from build123d import *

# Parameters (mm, degrees)
F0_W     = 2
F0_H     = 78
F1_DEPTH = 25
F0_W_2   = 16
F2_DEPTH = 2
F3_W     = 45.6874087788
F3_H     = 12.5
F4_DEPTH = 10
F7_DEPTH = 78
F8_DEPTH = 78


# Not quite as in the source:
# - a feature names something its author has since deleted; it is built from what else it names


with BuildPart() as f1:
    # F0 (on Top) → F1 (new body)
    with BuildSketch(Plane.XY):
        with Locations((9, 0)):
            Rectangle(F0_W, F0_H)
    extrude(amount=F1_DEPTH)



with BuildPart() as f1b:
    # F0 (on Top) → F1, piece 2 (new body)
    with BuildSketch(Plane.XY):
        with Locations((-9, 0)):
            Rectangle(F0_W, F0_H)
    extrude(amount=F1_DEPTH)


with BuildPart() as f1_1:
    add(f1.part)

    add(f1b.part)  # F2 merges F1b
    # F0 (on Top) → F2 (join)
    with BuildSketch(Plane.XY):
        with Locations((9, 0)):
            Rectangle(F0_W, F0_H)
        Rectangle(F0_W_2, F0_H)
        with Locations((-9, 0)):
            Rectangle(F0_W, F0_H)
    extrude(amount=F2_DEPTH)

    # F3 (on face) → F4 (cut)
    with BuildSketch(Plane(origin=(-10, 0, 0), x_dir=(0, -1, 0), z_dir=(-1, 0, 0))):
        with Locations((16.1562956106, 18.75)):
            Rectangle(F3_W, F3_H)
    extrude(amount=-F4_DEPTH, mode=Mode.SUBTRACT)

    # F6 (on face) → F7 (join)
    with BuildSketch(Plane(origin=(0, 39, 0), x_dir=(-1, 0, 0), z_dir=(0, 1, 0))):
        with BuildLine():
            ThreePointArc((-10, 7.8135579824), (-11.356996059, 3.1753555196), (-15, 0))
            Line((-15, 0), (-10, 0))
            Line((-10, 0), (-10, 7.8135579824))
        make_face()
    extrude(amount=-F7_DEPTH)

    # F5 (on face) → F8 (join)
    with BuildSketch(Plane(origin=(0, 39, 0), x_dir=(-1, 0, 0), z_dir=(0, 1, 0))):
        with BuildLine():
            Line((10, 0), (15, 0))
            ThreePointArc((15, 0), (11.360255444, 3.0951443467), (10, 7.6752495952))
            Line((10, 7.6752495952), (10, 0))
        make_face()
    extrude(amount=-F8_DEPTH)


solid = f1_1.part
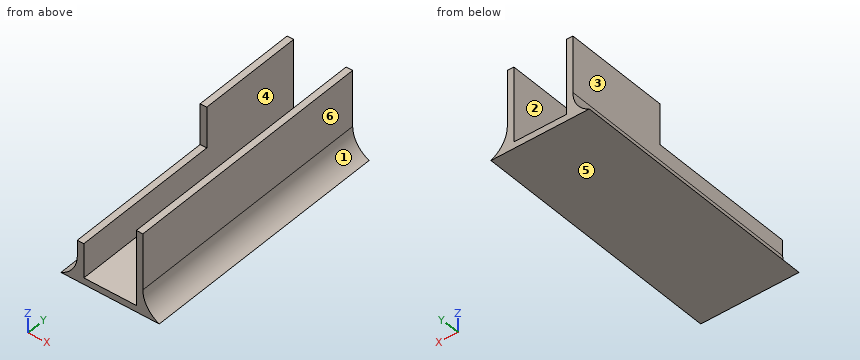
Could you check a few things on this model? Use its own coordinates, in mm. Face numbers are marked on the shaded views. A direction names the side the tool comes from. Coordinates: 2 decimals unless noted, no trailing zeros. Order: outer loops, then holes, each group sorted by start corner. A loop starts at its lowest first (then second) coordinate and runs counter-clockwise, first axis right, second up. Notation, with made-up numbers: (-27, -40) - (-3, -40) arc R31 ccw to (-3, -6) - close; hole circle Ø4 at (80.25, 27). An arc over 180 degrees is marked (long way). Answer in a Markdown table with one row per item. Add a question column.
(1) If we mould it in two halves opening along X, with no side actions, what happens to the marked faces 4, 5 and 6? For each: released by +X, released by -X, zero draft, split by the parting line, or undercut.
(2) I need wall thicknesses on L1, parallel to X at y = -1, z = 11.25; L2, parallel to Z at x = -6.75, y = -0.5; L3, parallel to X at y = -8, z = 13. Which ranges of each line are inside material? Lowest first, please.
(3) On a 3-axis mill with a long thin cutter (end or side, diameter ignored), from which of +Z, -Z, +X, -X, +Y, -Y can I reach the whole of each face in a straight line? I mean the marked faces 1, 2 and 3. Say none if no direction works.
(4) If we section it at D-D, the plane z = 11.5: Please give me the cut outline in (x, y), then the cut area to 3 significant figures.
(5) If we section it at B-B, the plane y = -21.5: Please give me the cut outline in (x, z).
(6) If we section it at C-C, the plane x = -4.5: Please give me the cut outline in (y, z).
(7) If we section it at A-A, the plane z = 15.25: Please give me the cut outline in (x, y), then the cut area to 3 significant figures.
(8) Will these pins go through, and if not, where does the flat tip stop? pin 1 (1.5 mm diameter, centred on y = -26.5, z = 19.5, fed in from +X); pin 2 (0.6 mm diameter, centred on x = -9.5, y = -9, fed in from +Z); pin 3 (5 mm diameter, centred on y = 17.5, z = 18, fed in from -X).
Results are:
| question | item | result |
|---|---|---|
| 1 | face 4 | undercut |
| 1 | face 5 | zero draft |
| 1 | face 6 | released by +X |
| 2 | L1 | x = -10 to -8, 8 to 10 |
| 2 | L2 | z = 0 to 2 |
| 2 | L3 | x = 8 to 10 |
| 3 | face 1 | +Z, +X, +Y, -Y |
| 3 | face 2 | +Z, +Y, -Y |
| 3 | face 3 | +Z, -X, +Y, -Y |
| 4 | outline | (-10, -39) - (-8, -39) - (-8, 39) - (-10, 39) - close; (8, -39) - (10, -39) - (10, 39) - (8, 39) - close |
| 4 | area | 312 mm2 |
| 5 | outline | (-15, 0) - (15, 0) arc R8.61 cw to (10, 7.81) - (10, 25) - (8, 25) - (8, 2) - (-8, 2) - (-8, 12.5) - (-10, 12.5) - (-10, 7.68) arc R8.39 cw to start |
| 6 | outline | (-39, 0) - (39, 0) - (39, 2) - (-39, 2) - close |
| 7 | outline | (-10, 6.69) - (-8, 6.69) - (-8, 39) - (-10, 39) - close; (8, -39) - (10, -39) - (10, 39) - (8, 39) - close |
| 7 | area | 221 mm2 |
| 8 | pin 1 | stops at x = 10 |
| 8 | pin 2 | stops at z = 12.5 |
| 8 | pin 3 | stops at x = -10 |
